from build123d import *

# Parameters (mm, degrees)
F0_R            = 11
F1_DEPTH        = 4
F3_DEPTH        = 4.001
F3_COPIES_COUNT = 12
F5_R            = 3.15
F6_DEPTH        = 3
F7_W            = 3.6
F7_H            = 3.6
F8_DEPTH        = 7


# Not quite as in the source:
# - a pattern or mirror of a feature is missing from the dataset's text; its kind, count and spacing are read off the source's solid


with BuildPart() as f1:
    # F0 (on Top) → F1 (new body)
    with BuildSketch(Plane.XY):
        Circle(F0_R)
    extrude(amount=F1_DEPTH)

    # F2 (on face) → F3 (cut, through all)
    with BuildSketch(Plane.XY.offset(4)):
        with BuildLine():
            ThreePointArc((-0.2442964769, 6.9957357891), (-0.1221668451, 6.9989338661), (0, 7))
            Line((0, 7), (0, 11))
            ThreePointArc((0, 11), (-1.2452353514, 10.9292904124), (-2.4744615978, 10.7180707126))
            Line((-2.4744615978, 10.7180707126), (-0.2442964769, 6.9957357891))
        make_face()
        with BuildLine():
            Line((0, 11), (0, 7))
            ThreePointArc((0, 7), (0.1221668451, 6.9989338661), (0.2442964769, 6.9957357891))
            Line((0.2442964769, 6.9957357891), (2.4744615978, 10.7180707126))
            ThreePointArc((2.4744615978, 10.7180707126), (1.2452353514, 10.9292904124), (0, 11))
        make_face()
    f3 = extrude(amount=-F3_DEPTH, mode=Mode.SUBTRACT)

    # F3_copies: F3 ×12 about axis
    f3_copies_axis = Axis((0, 0, 0), (0, 0, 1))
    for i in range(1, F3_COPIES_COUNT):
        add(f3.rotate(f3_copies_axis, i * 360 / F3_COPIES_COUNT), mode=Mode.SUBTRACT)

    # F5 (on face) → F6 (join)
    with BuildSketch(Plane.XY.offset(4)):
        Circle(F5_R)
    extrude(amount=F6_DEPTH)

    # F7 (on face) → F8 (cut, through all)
    with BuildSketch(Plane.XY.offset(7)):
        Rectangle(F7_W, F7_H)
    extrude(amount=-F8_DEPTH, mode=Mode.SUBTRACT)


solid = f1.part
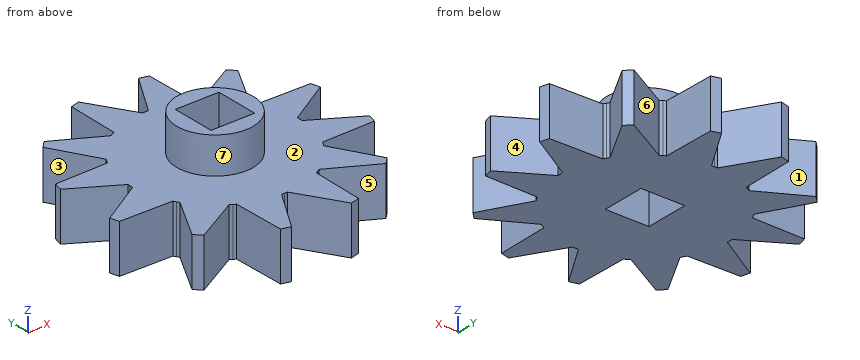
Check sheet for the modelled part. Datum: model origin and axes. Units: mm. Face numbers are marked on the shaded views. A direction names the side the tool comes from. Give positions to 0.01 mm unless a question says otherwise; leave off trailing zeros. Loops run counter-clockwise (first coordinate to the right, second up) from the corner with the lowest first, then second, coordinate; pieces in that order, holes last. Notation, with made-up numbers: M 34.5,-30.5 L 47.5,-30.5 A6 cw 47.5,-26.5 Z; hole C 29,9.5 d9. An arc over 180 degrees is marked long. Use a Markdown table: item, result. Add a question column.
Q1. Scan lines: line 1 along X through (y, z) = (-6.25, 2); line 2 along Z through (x, y) = (2.5, -6.25); line 3 along Y through (x, z) = (9.25, 1.25). Record each from-to range of solid material in increasing order. Write a range as [from, to].
Q2. Sectioned sample at C-C, the plane y = -8.5. Record the cut outline in (x, z).
Q3. Go/stop test with flat-tipped pins: pin 1 (4 mm diameter, centred on x = -4.5, z = 4.5, fed in from +Y); pin 2 (4 mm diameter, centred on x = -0.5, y = 7, fed in from +Z); pin 3 (3 mm diameter, centred on x = -0.5, z = 3, fed in from -Y). Record where each tip stops, or that it passes through.
Q4. Tool access check on the marked faces 4, 5, 6 and 7. Record the directions out of +Z, -Z, +X, -X, +Y, -Y that give a thin tool (end or side, any length) a straight path to the whole face; none if there is none.
Q5. Mould release check, pull along Y, two halves, no side actions. Record for the marked faces 1, 2 and 3: pulls with the +Y half, pulls with the -Y half, needs draft (parallel to the pull), parting line crosses it, or undercut.
Q6. Sectioned sample at A-A, the plane x = 1.25. Record the cut outline in (y, z).
Q7. Sectioned sample at D-D, the plane y = 4.5. Record the cut outline in (x, z).
Q8. Sectioned sample at B-B, the plane z = 5. Record the cut outline in (x, y), then the cut area to 3 significant figures.
Verdict:
| question | item | result |
|---|---|---|
| 1 | line 1 | [-7.35, -4.27], [-3.29, 3.29], [4.27, 7.35] |
| 1 | line 2 | [0, 4] |
| 1 | line 3 | [-3.24, -1.59], [1.59, 3.24] |
| 2 | outline | M -3.25,0 L -1.15,0 L -1.15,4 L -3.25,4 Z; M 1.15,0 L 3.25,0 L 3.25,4 L 1.15,4 Z |
| 3 | pin 1 | y = 10.7 |
| 3 | pin 2 | z = 4 |
| 3 | pin 3 | y = -9.93 |
| 4 | face 4 | +Z, -Z, +X |
| 4 | face 5 | +Z, -Z, -Y |
| 4 | face 6 | +Z, -Z, +Y |
| 4 | face 7 | +Z |
| 5 | face 1 | pulls with the +Y half |
| 5 | face 2 | needs draft |
| 5 | face 3 | undercut |
| 6 | outline | M -8.67,0 L -1.8,0 L -1.8,7 L -2.89,7 L -2.89,4 L -8.67,4 Z; M 1.8,0 L 8.67,0 L 8.67,4 L 2.89,4 L 2.89,7 L 1.8,7 Z |
| 7 | outline | M -6.38,0 L 6.38,0 L 6.38,4 L -6.38,4 Z |
| 8 | outline | C 0,0 d6.3; hole M -1.8,-1.8 L 1.8,-1.8 L 1.8,1.8 L -1.8,1.8 Z |
| 8 | area | 18.2 mm^2 |
